```python
from build123d import *

# Parameters (mm, degrees)
F0_R     = 1.5
F0_W     = 3
F0_H     = 20
F1_DEPTH = 3
F3_DEPTH = 25


with BuildPart() as f1:
    # F0 (on Top) → F1 (new body)
    with BuildSketch(Plane.XY):
        with BuildLine():
            Line((-7.5, 25), (-7.5, 0))
            Line((-7.5, 0), (-6, 0))
            Line((-6, 0), (-6, -5))
            ThreePointArc((-6, -5), (-4.535534, -8.535534), (-1, -10))
            Line((-1, -10), (1, -10))
            ThreePointArc((1, -10), (4.535534, -8.535534), (6, -5))
            Line((6, -5), (6, 0))
            Line((6, 0), (7.5, 0))
            Line((7.5, 0), (7.5, 25))
            Line((7.5, 25), (6, 28))
            Line((6, 28), (-6, 28))
            Line((-6, 28), (-7.5, 25))
        make_face()
        with Locations((0, -5)):
            Circle(F0_R, mode=Mode.SUBTRACT)
        with Locations((0, 13)):
            Rectangle(F0_W, F0_H, mode=Mode.SUBTRACT)
    extrude(amount=F1_DEPTH)

    # F2 (on face) → F3 (cut)
    with BuildSketch(Plane(origin=(0, 0, 0), x_dir=(1, 0, 0), z_dir=(0, 0, -1))):
        Polygon((-6.98, -0.976704), (-4.143444, 0), (-6, 0), (-7.5, 0), (-7.5, -25), (-4.143444, -23.55), (-4.143444, -22.378409), (-6.98, -21.401704), (-6.98, -20.601704), (-4.143444, -19.625), (-4.143444, -18.453409), (-6.98, -17.476704), (-6.98, -16.676704), (-4.143444, -15.7), (-4.143444, -14.528409), (-6.98, -13.551704), (-6.98, -12.751704), (-4.143444, -11.775), (-4.143444, -10.603409), (-6.98, -9.626704), (-6.98, -8.826704), (-4.143444, -7.85), (-4.143444, -6.678409), (-6.98, -5.701704), (-6.98, -4.901704), (-4.143444, -3.925), (-4.143444, -2.753409), (-6.98, -1.776704), align=None)
        Polygon((4.143444, -23.55), (7.5, -25), (7.5, 0), (6, 0), (4.143444, 0), (6.98, -0.976704), (6.98, -1.776704), (4.143444, -2.753409), (4.143444, -3.925), (6.98, -4.901704), (6.98, -5.701704), (4.143444, -6.678409), (4.143444, -7.85), (6.98, -8.826704), (6.98, -9.626704), (4.143444, -10.603409), (4.143444, -11.775), (6.98, -12.751704), (6.98, -13.551704), (4.143444, -14.528409), (4.143444, -15.7), (6.98, -16.676704), (6.98, -17.476704), (4.143444, -18.453409), (4.143444, -19.625), (6.98, -20.601704), (6.98, -21.401704), (4.143444, -22.378409), align=None)
    extrude(amount=-F3_DEPTH, mode=Mode.SUBTRACT)


solid = f1.part
```
For this review, take the finished solid that the model builds, in its own axes (mm). A direction names the side the tool comes from. Round coordinates to 2 decimals unless told otherwise and drop trailing zeros. Order: outer loops, then holes, each group sorted by start corner. A loop starts at its lowest first (then second) coordinate and runs counter-clockwise, first axis right, second up.
Q1. We need section B-B, the plane y = 18. Give the boundary of the cut face in (x, z), plus the area to 3 significant figures.
Findings below:
outline: (-5.46, 0) - (-1.5, 0) - (-1.5, 3) - (-5.46, 3) - close; (1.5, 0) - (5.46, 0) - (5.46, 3) - (1.5, 3) - close
area: 23.8 mm2
Q2. We need section A-A, the plane x = 0. Give the boundary of the cut face in (y, z).
Findings below:
outline: (-10, 0) - (-6.5, 0) - (-6.5, 3) - (-10, 3) - close; (-3.5, 0) - (3, 0) - (3, 3) - (-3.5, 3) - close; (23, 0) - (28, 0) - (28, 3) - (23, 3) - close
Q3. Mouldability with a two-part tool opening along Y and no side actions: class faces 1 (the cylindrical face through (4, -9, 1)), 2 (the flat face through (-4.143, 19, 1)), 3 (the flat face through (6.98, 1.4, 1.5)) as pulls with the +Y half, pulls with the -Y half, needs draft (parallel to the pull), parting line crosses it, or undercut.
Findings below:
face 1: pulls with the -Y half
face 2: undercut
face 3: needs draft
Q4. Insertion check: P1, Ø2, axis at x = 4, y = 4, coming from the -Z side; P2, Ø1.5, axis at y = -3.5, z = 1, coming from the +X side; P3, Ø1.3, axis at y = 23, z = 1.5, coming from the -X side; P4, Ø0.9, axis at y = 17, z = 1.5, coming from the +X side. Each pin has a flat end and moves straight along its axis. Give the tip position at first contact, or say it passes through.
Findings below:
P1: stops at z = 0
P2: stops at x = 6
P3: stops at x = -4.37
P4: stops at x = 6.98
Q5. Wall thickness on line 1 (Y direction, x = 0, z = 0.8); line 2 (X direction, y = 19, z = 1.85); line 3 (Y direction, x = -0.5, z = 0.3): over which ranges is each line inside the solid? List them lowest first.
Findings below:
line 1: y = -10 to -6.5, -3.5 to 3, 23 to 28
line 2: x = -4.14 to -1.5, 1.5 to 4.14
line 3: y = -10 to -6.41, -3.59 to 3, 23 to 28
Q6. Machinability: for faces 4 (the flat face through (-6.98, 1.4, 1.5)), 5 (the flat face through (0, -10, 1)), 6 (the flat face through (5.6, 10.1, 1.5)), 7 (the flat face through (-4.143, 7, 1)), 8 (the cylindrical face through (-0.195, -3.513, 1.479)), which of the approach directions +Z, -Z, +X, -X, +Y, -Y give a long, thin tool a straight path to every point of the face, cutting with its end or side? Answer none if there is none.
Findings below:
face 4: +Z, -Z, -X, -Y
face 5: +Z, -Z, +X, -X, -Y
face 6: +Z, -Z, +X
face 7: +Z, -Z, -X
face 8: +Z, -Z
Q7. We need section C-C, the plane x = -5.25. State how many separate pieces and enclosed holes the cut face has, plus the area to 3 significant figures.
Findings below:
separate pieces: 8
enclosed holes: 0
area: 70.7 mm2
